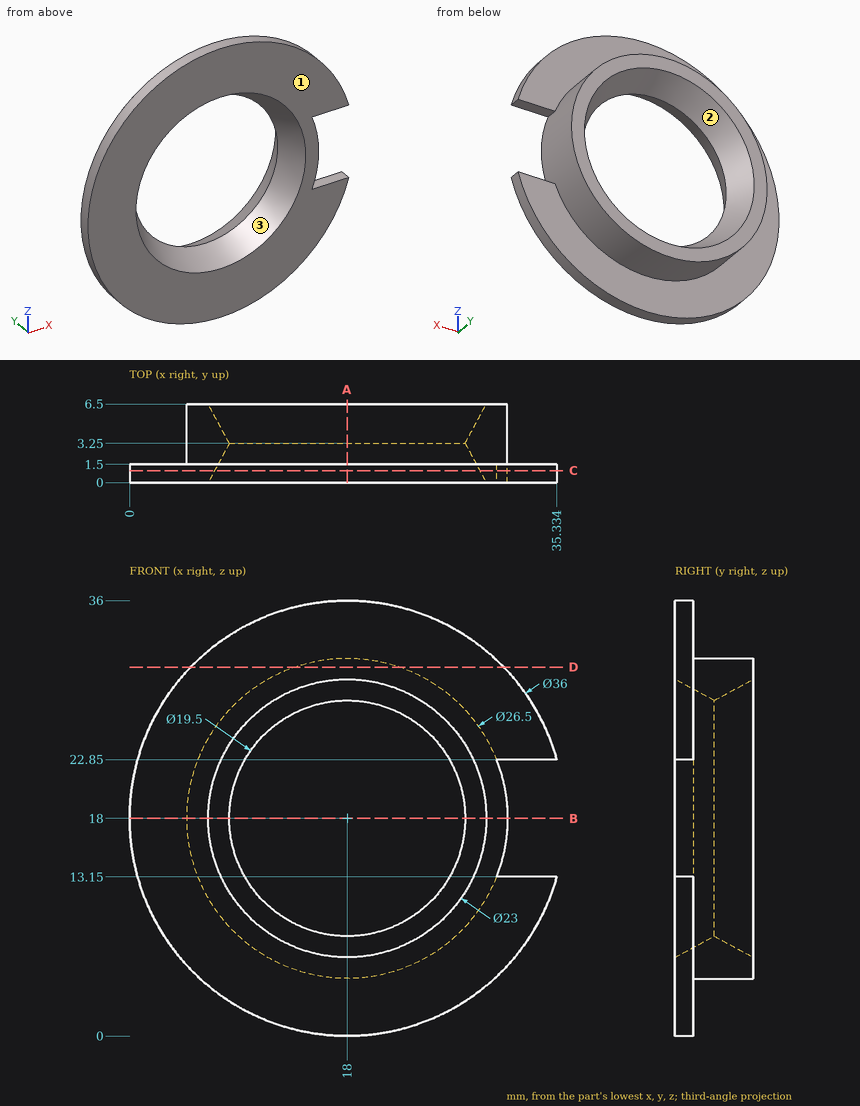
Can you work these out from the drawing? Everything is in mm from the part's minimum corner. Coordinates: 2 decimals unless noted, no trailing zeros. Write each loop counter-clockwise with the first axis right and the second up, starting at its lowest first coordinate (ties: lowest second). Pieces come first, ordered by that corner, then holes. Notation, with made-up numbers: (18.25, -4.5) -> (37.25, -4.5) arc R15 ccw to (37.25, 19.5) -> close; hole circle Ø3 at (34, 66). An arc over 180 degrees is marked (long way). Return JSON: item names as keys, results as strings.
(1) Imagine slicing it at C-C, the plane y = 1. Please give me the cut outline in (x, z).
Numbers:
{"outline": "(30.33, 13.15) arc R13.25 ccw to (30.33, 22.85) -> (35.33, 22.85) arc R18 ccw (long way) to (35.33, 13.15) -> close; hole circle Ø21.92 at (18, 18)"}
(2) Imagine slicing it at A-A, the plane x = 18. Please give me the cut outline in (y, z).
Numbers:
{"outline": "(0, 0) -> (1.5, 0) -> (1.5, 4.75) -> (6.5, 4.75) -> (6.5, 6.5) -> (3.25, 8.25) -> (0, 6.5) -> close; (0, 29.5) -> (3.25, 27.75) -> (6.5, 29.5) -> (6.5, 31.25) -> (1.5, 31.25) -> (1.5, 36) -> (0, 36) -> close"}
(3) Imagine slicing it at D-D, the plane z = 30.5. Please give me the cut outline in (x, y) (1 decimal), then the cut area to 3 significant figures.
Numbers:
{"outline": "(5, 0) -> (31, 0) -> (31, 1.5) -> (22.4, 1.5) -> (22.4, 6.5) -> (13.6, 6.5) -> (13.6, 1.5) -> (5, 1.5) -> close", "area": "82.8 mm2"}
(4) I'm going to push flat-ended pins straight in: pin 1 (3 mm diameter, centred on x = 19.5, y = 2.5, fed in from -Z); pin 2 (1.2 mm diameter, centred on x = 31.5, y = 0.5, fed in from +Z). Where does each tip first touch, or does it pass through?
Numbers:
{"pin 1": "stops at z = 0", "pin 2": "stops at z = 30.55"}
(5) Imagine slicing it at B-B, the plane z = 18. Please give me the cut outline in (x, y).
Numbers:
{"outline": "(0, 0) -> (6.5, 0) -> (8.25, 3.25) -> (6.5, 6.5) -> (4.75, 6.5) -> (4.75, 1.5) -> (0, 1.5) -> close; (27.75, 3.25) -> (29.5, 0) -> (31.25, 0) -> (31.25, 6.5) -> (29.5, 6.5) -> close"}
(6) I need wall thicknesses on L1, parallel to Z at x = 21, y = 4.25 (1 decimal); L2, parallel to X at y = 3.75, z = 10.5 (1 decimal); L3, parallel to Y at x = 2, z = 16.5. Which ranges of each line are inside material? Lowest first, please.
Numbers:
{"L1": "z = 5.1 to 8.2, 27.8 to 30.9", "L2": "x = 7.1 to 11.4, 24.6 to 28.9", "L3": "y = 0 to 1.5"}
(7) We'd pull the mould along X, two halves only. Please class the marked faces 1, 2 and 3: +X half, -X half, draft (parallel to the pull), parting line (faces both ways), or undercut.
Numbers:
{"face 1": "draft", "face 2": "undercut", "face 3": "undercut"}
